Input: dimensioned drawing with shaded views. Units: mm. Origin: part minimum x, y, z. Coordinates: 2 decimals unless noted, no trailing zeros. Loops run counter-clockwise (first coordinate to the right, second up) from the corner with the lowest first, then second, coordinate; pieces in that order, holes last.
Item 1: Pull-direction query (Y, two-part tool) for the marked faces 1, 2 and 3; classes: +Y half, -Y half, draft (parallel to the pull), parting line (faces both ways), or undercut.
Item 2: Section query B-B, the plane z = 4.5. Return the cut outline in (x, y), then the cut area to 3 significant figures.
Item 3: Line query: probe 1 along Y at (x, z) = (23, 19); probe 2 along X at (y, z) = (2.5, 15.5); probe 3 along Z at (x, y) = (8, 2.25). Output: solid intervals per line, ascending.
Item 4: Pin query (flat end, axial travel): pin 1 Ø7.5 at (x, z) = (10.5, 9) entering from -Y. Return the tip coordinate at first contact, or that it passes through.
Item 5: Section query A-A, the plane x = 12.7. Return the cut outline in (y, z), then the cut area to 3 significant figures.
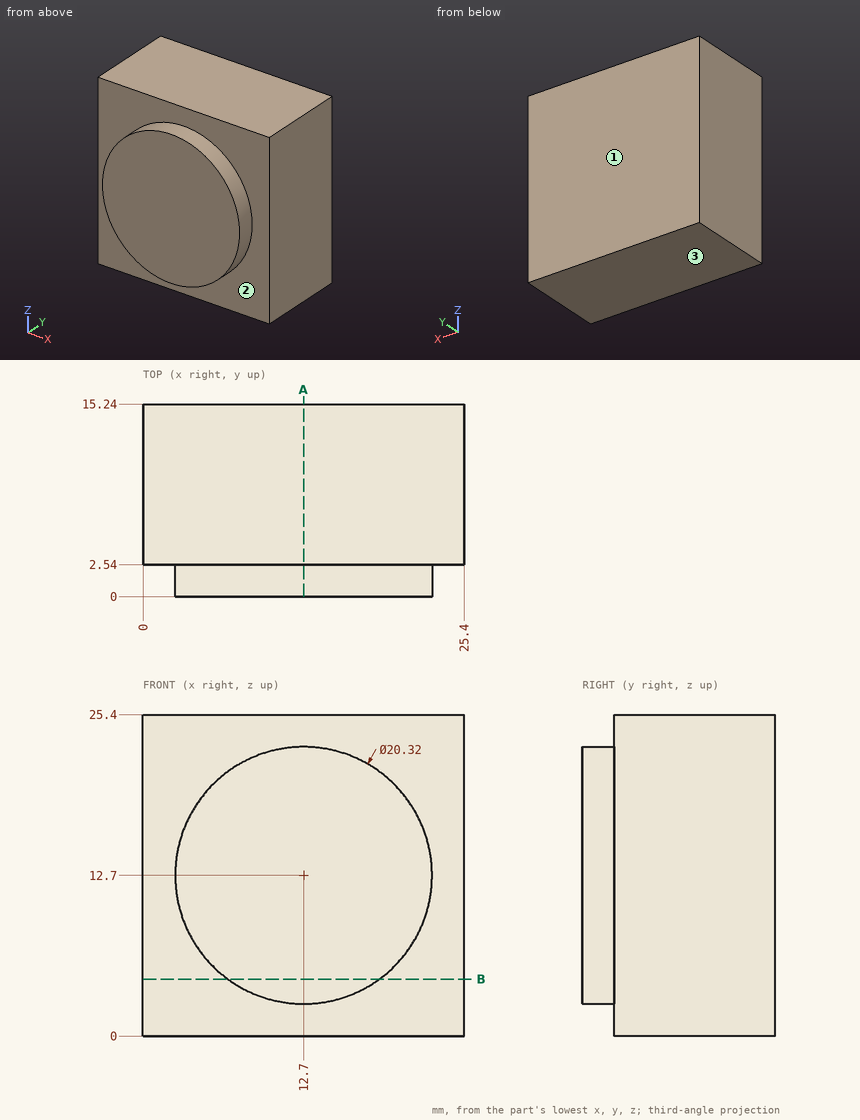
Verdict:
1. face 1: +Y half
1. face 2: -Y half
1. face 3: draft
2. outline: (0, 2.54) - (6.7, 2.54) - (6.7, 0) - (18.7, 0) - (18.7, 2.54) - (25.4, 2.54) - (25.4, 15.24) - (0, 15.24) - close
2. area: 353 mm2
3. probe 1: y = 2.54 to 15.24
3. probe 2: x = 2.93 to 22.47
3. probe 3: z = 3.69 to 21.71
4. pin 1: stops at y = 0
5. outline: (0, 2.54) - (2.54, 2.54) - (2.54, 0) - (15.24, 0) - (15.24, 25.4) - (2.54, 25.4) - (2.54, 22.86) - (0, 22.86) - close
5. area: 374 mm2
